Part model, mm, in its own coordinate system. A direction names the side the tool comes from. Round coordinates to 2 decimals unless told otherwise and drop trailing zeros. Use a Markdown table: item, result. Add a question column.
Item 1: Probe line 1 (Y direction, x = 144, z = -2.6) (3 decimals). List the from-to ranges inside material, lowest first. Write a range as [from, to].
Item 2: Cut at A-A, the plane y = 2.05. State how many separate pieces and enclosed holes the cut face has, plus the area to 3 significant figures.
Item 3: Which spindle directions (+Z, -Z, +X, -X, +Y, -Y) get a long thin tool onto all of the face, cutting with end or side? Do faces 1 (the face through (72, 1, 0)), 2 (the face through (-3, 0.875, -2)), 3 (the face through (150, 0.875, -2)). Say none if no direction does.
Item 4: Flat gauge pin, fed straight in: pin 1 (0.6 mm diameter, centred on x = 73.5, z = -1.5, fed in from +Y) (3 decimals). Where does the tip first touch, or does it go through?
```python
from build123d import *

# Parameters (mm, degrees)
BLANKSKE_W          = 147
BLANKSKE_H          = 2.9
BLANK_DEPTH         = 4.5
TOOTHCUTSIM_DEPTH   = 148.097450692
TEETHCUTS_COUNT     = 53
TEETHCUTS_PITCH     = 2.827433385
SKETCH1_W           = 4.5
SKETCH1_H           = 0.875
BOSS_EXTRUDE1_DEPTH = 6
SKETCH2_W           = 4.5
SKETCH2_H           = 0.875
BOSS_EXTRUDE2_DEPTH = 6
SKETCH3_W           = 159
SKETCH3_H           = 4.5
BOSS_EXTRUDE3_DEPTH = 1


with BuildPart() as part:
    # BlankSke → Blank (new body)
    with BuildSketch(Plane.XY):
        with Locations((73.5, 1.45)):
            Rectangle(BLANKSKE_W, BLANKSKE_H)
    extrude(amount=-BLANK_DEPTH)

    # TooCutSkeSim → ToothCutSim (cut, through all)
    with BuildSketch(Plane.XY):
        Polygon((0.399391833, 0.875), (-0.399391833, 0.875), (-1.145676401, 2.9254), (1.145676401, 2.9254), align=None)
    toothcutsim = extrude(amount=-TOOTHCUTSIM_DEPTH, mode=Mode.SUBTRACT)

    # TeethCuts: ToothCutSim ×53
    with Locations(*[(i * TEETHCUTS_PITCH, 0, 0) for i in range(1, TEETHCUTS_COUNT)]):
        add(toothcutsim, mode=Mode.SUBTRACT)

    # Sketch1 → Boss-Extrude1 (add)
    with BuildSketch(Plane(origin=(147, 0, 0), x_dir=(0, 0, -1), z_dir=(1, 0, 0))):
        with Locations((2.25, 0.4375)):
            Rectangle(SKETCH1_W, SKETCH1_H)
    extrude(amount=BOSS_EXTRUDE1_DEPTH)

    # Sketch2 → Boss-Extrude2 (add)
    with BuildSketch(Plane.ZY):
        with Locations((-2.25, 0.4375)):
            Rectangle(SKETCH2_W, SKETCH2_H)
    extrude(amount=BOSS_EXTRUDE2_DEPTH)

    # Sketch3 → Boss-Extrude3 (add)
    with BuildSketch(Plane.XZ):
        with Locations((73.5, -2.25)):
            Rectangle(SKETCH3_W, SKETCH3_H)
    extrude(amount=BOSS_EXTRUDE3_DEPTH)


solid = part.part
```
A:
| question | item | result |
|---|---|---|
| 1 | line 1 | y = [-1, 0.875] |
| 2 | separate pieces | 52 |
| 2 | enclosed holes | 0 |
| 2 | area | 275 mm^2 |
| 3 | face 1 | +Z, +X, -X, +Y, -Y |
| 3 | face 2 | +Z, -Z, -X, +Y |
| 3 | face 3 | +Z, -Z, +X, +Y |
| 4 | pin 1 | stops at y = 0.875 |
